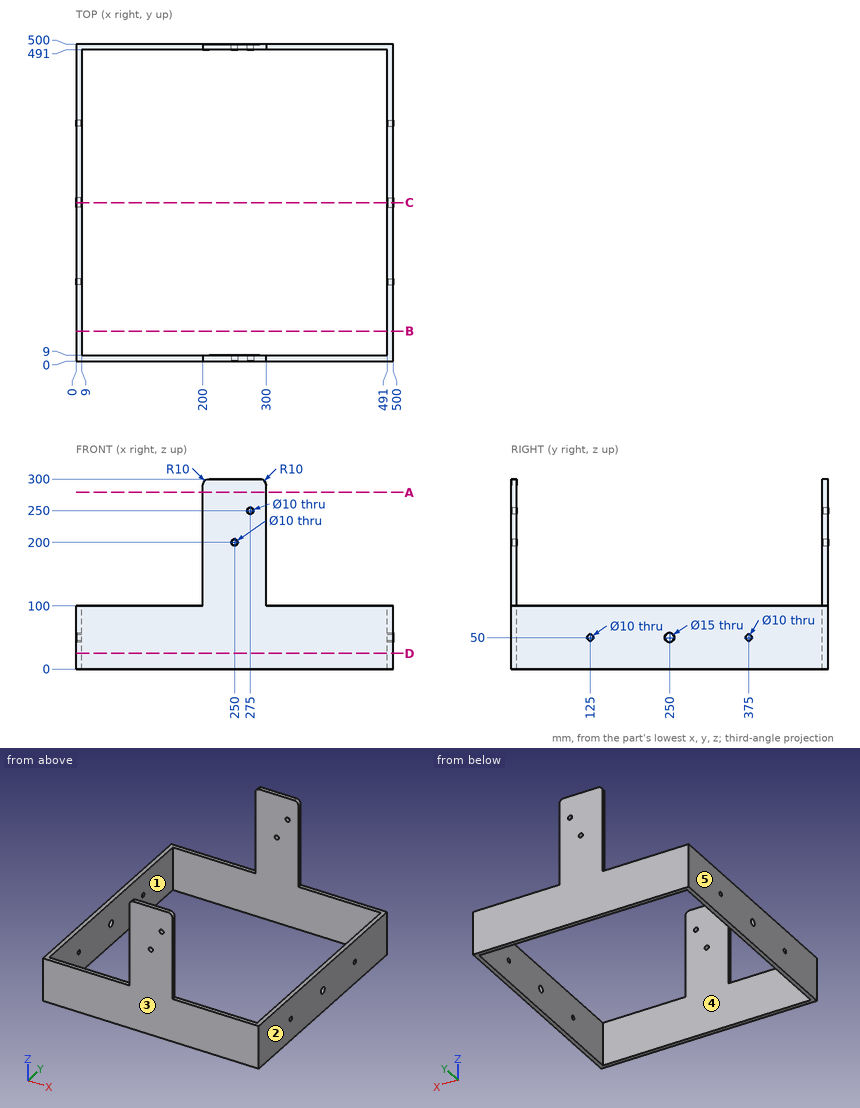
Drawing for the job (mm, zero at the part's lowest x, y, z). A direction names the side the tool comes from. Give positions to 0.01 mm unless a question says otherwise; leave off trailing zeros. Loops run counter-clockwise (first coordinate to the right, second up) from the corner with the lowest first, then second, coordinate; pieces in that order, holes last. Notation, with made-up numbers: M 61.5,26.5 L 78.5,26.5 A21 cw 78.5,48.5 Z; hole C 49.5,73 d7. An arc over 180 degrees is marked long. Use one line per item in the form item = value.
Item 1: Flat gauge pins, fed straight in: pin 1 (8 mm diameter, centred on y = 67.5, z = 99, fed in from -X); pin 2 (10 mm diameter, centred on y = 493.5, z = 219, fed in from +X); pin 3 (6 mm diameter, centred on y = 125, z = 50, fed in from -X). Where does each tip first touch, or does it go through?
Determined:
pin_1 = 0
pin_2 = 300
pin_3 = through
Item 2: Slice it at D-D (z = 25). List the corners of the cut face in (x, y).
Determined:
outline = M 0,0 L 500,0 L 500,500 L 0,500 Z; hole M 9,9 L 491,9 L 491,491 L 9,491 Z
Item 3: Slice it at A-A (z = 279). List the corners of the cut face in (x, y).
Determined:
outline = M 200,0 L 300,0 L 300,9 L 200,9 Z; M 200,491 L 300,491 L 300,500 L 200,500 Z
Item 4: Slice it at B-B (y = 47). List the corners of the cut face in (x, z).
Determined:
outline = M 0,0 L 9,0 L 9,100 L 0,100 Z; M 491,0 L 500,0 L 500,100 L 491,100 Z
Item 5: Drill centre lines: probe 1 along Y at (x, z) = (493.5, 50); probe 2 along X at (y, z) = (495, 200); probe 3 along X at (y, z) = (467, 74.5). Where is each one in solid material? Low to high. Write a range as from..to.
Determined:
probe_1 = 0..120, 130..242.5, 257.5..370, 380..500
probe_2 = 200..245, 255..300
probe_3 = 0..9, 491..500
Item 6: Which spindle directions (+Z, -Z, +X, -X, +Y, -Y) get a long thin tool onto all of the face, cutting with end or side? Do the marked faces 1 and 2. Say none if no direction does.
Determined:
face_1 = +Z, -Z
face_2 = +Z, -Z, +X, +Y, -Y
Item 7: Slice it at C-C (y = 250). List the corners of the cut face in (x, z).
Determined:
outline = M 0,0 L 9,0 L 9,42.5 L 0,42.5 Z; M 0,57.5 L 9,57.5 L 9,100 L 0,100 Z; M 491,0 L 500,0 L 500,42.5 L 491,42.5 Z; M 491,57.5 L 500,57.5 L 500,100 L 491,100 Z
Item 8: Two-plate mould, pull along X, no slides. Class the marked faces 3, 4 and 5: pulls with the +X half, pulls with the -X half, needs draft (parallel to the pull), parting line crosses it, or undercut.
Determined:
face_3 = needs draft
face_4 = undercut
face_5 = pulls with the -X half
